from build123d import *

# Parameters (mm, degrees)
F0_W      = 1219.2
F0_H      = 50.8
F1_DEPTH  = 609.6
F3_R      = 10.16
F4_R      = 10.16
F5_R      = 10.16
F6_R      = 10.16
F7_R      = 5.08
F8_W      = 63.5
F8_H      = 63.5
F9_DEPTH  = 457.2
F10_R     = 7.62
F11_W     = 63.5
F11_H     = 63.5
F12_DEPTH = 457.2
F13_R     = 7.62
F14_W     = 63.5
F14_H     = 63.5
F15_DEPTH = 457.2
F16_R     = 7.62
F17_W     = 63.5
F17_H     = 63.5
F18_DEPTH = 457.2
F19_R     = 7.62


with BuildPart() as f1:
    # F0 (on Front) → F1 (new body)
    with BuildSketch(Plane.XZ):
        Rectangle(F0_W, F0_H)
    extrude(amount=F1_DEPTH)

    # F3
    f3_edges = [f1.edges().sort_by_distance(p)[0] for p in [
        (-609.6, -609.6, 0),
    ]]
    fillet(f3_edges, radius=F3_R)

    # F4
    f4_edges = [f1.edges().sort_by_distance(p)[0] for p in [
        (-609.6, 0, 0),
    ]]
    fillet(f4_edges, radius=F4_R)

    # F5
    f5_edges = [f1.edges().sort_by_distance(p)[0] for p in [
        (609.6, 0, 0),
    ]]
    fillet(f5_edges, radius=F5_R)

    # F6
    f6_edges = [f1.edges().sort_by_distance(p)[0] for p in [
        (609.6, -609.6, 0),
    ]]
    fillet(f6_edges, radius=F6_R)

    # F7
    f7_edges = [f1.edges().sort_by_distance(p)[0] for p in [
        (-609.6, -304.8, 25.4),
        (-609.6, -304.8, -25.4),
    ]]
    fillet(f7_edges, radius=F7_R)

    # F8 (on face) → F9 (join)
    with BuildSketch(Plane(origin=(0, 0, -25.4), x_dir=(1, 0, 0), z_dir=(0, 0, -1))):
        with Locations((-538.884262, 70.392589)):
            Rectangle(F8_W, F8_H)
    extrude(amount=F9_DEPTH)

    # F10
    f10_edges = [f1.edges().sort_by_distance(p)[0] for p in [
        (-507.134262, -38.642589, -254),
        (-507.134262, -102.142589, -254),
        (-570.634262, -102.142589, -254),
        (-570.634262, -38.642589, -254),
    ]]
    fillet(f10_edges, radius=F10_R)

    # F11 (on face) → F12 (join)
    with BuildSketch(Plane(origin=(0, 0, -25.4), x_dir=(1, 0, 0), z_dir=(0, 0, -1))):
        with Locations((533.460811, 75.974436)):
            Rectangle(F11_W, F11_H)
    extrude(amount=F12_DEPTH)

    # F13
    f13_edges = [f1.edges().sort_by_distance(p)[0] for p in [
        (565.210811, -107.724436, -254),
        (565.210811, -44.224436, -254),
        (501.710811, -107.724436, -254),
        (501.710811, -44.224436, -254),
    ]]
    fillet(f13_edges, radius=F13_R)

    # F14 (on face) → F15 (join)
    with BuildSketch(Plane(origin=(0, 0, -25.4), x_dir=(1, 0, 0), z_dir=(0, 0, -1))):
        with Locations((-538.621542, 539.01282)):
            Rectangle(F14_W, F14_H)
    extrude(amount=F15_DEPTH)

    # F16
    f16_edges = [f1.edges().sort_by_distance(p)[0] for p in [
        (-570.371542, -570.76282, -254),
        (-506.871542, -570.76282, -254),
        (-506.871542, -507.26282, -254),
        (-570.371542, -507.26282, -254),
    ]]
    fillet(f16_edges, radius=F16_R)

    # F17 (on face) → F18 (join)
    with BuildSketch(Plane(origin=(0, 0, -25.4), x_dir=(1, 0, 0), z_dir=(0, 0, -1))):
        with Locations((538.63135, 542.144825)):
            Rectangle(F17_W, F17_H)
    extrude(amount=F18_DEPTH)

    # F19
    f19_edges = [f1.edges().sort_by_distance(p)[0] for p in [
        (570.38135, -573.894825, -254),
        (506.88135, -573.894825, -254),
        (506.88135, -510.394825, -254),
        (570.38135, -510.394825, -254),
    ]]
    fillet(f19_edges, radius=F19_R)


solid = f1.part
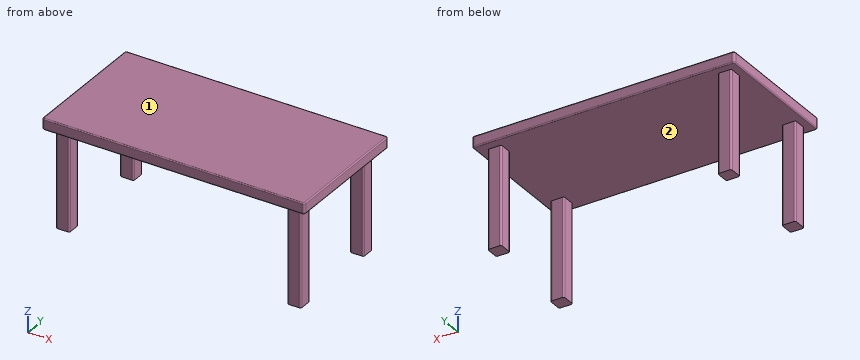
Part model, mm, in its own coordinate system. Face numbers are marked on the shaded views. A direction names the side the tool comes from. Coordinates: 2 decimals unless noted, no trailing zeros. Write each loop counter-clockwise with the first axis right and the second up, starting at its lowest first coordinate (ties: lowest second). Pieces come first, ordered by that corner, then holes. Notation, with made-up numbers: (11, -8.5) - (43, -8.5) arc R22 cw to (43, 12.5) - close; hole circle Ø2 at (35.25, 89). An arc over 180 degrees is marked (long way). Put each result on its own line as item: value.
1. Band-saw the part on A-A (z = -155.5). Give the number of separate pieces and of enclosed holes in the cut face, then the cut area to 3 significant figures.
Final values:
separate pieces: 4
enclosed holes: 0
area: 15,900 mm²
2. Flat gauge pins, fed straight in: pin 1 Ø14.5 at (x, z) = (546.5, -329) entering from -Y; pin 2 Ø24 at (x, z) = (521.5, -150) entering from +Y; pin 3 Ø14.5 at (y, z) = (-77.5, -307.5) entering from -X; pin 4 Ø10 at (y, z) = (-501, -238) entering from -X. Where does each tip first touch, or does it go through?
Final values:
pin 1: stops at y = -573.89
pin 2: stops at y = -44.22
pin 3: stops at x = -570.63
pin 4: passes through
3. 3-axis set-ups, long thin cutter, end or side, ignore diameter. For the marked faces 1 and 2: which of +Z, -Z, +X, -X, +Y, -Y reach the whole face in a straight line?
Final values:
face 1: +Z, +X, -X, +Y, -Y
face 2: -Z
4. Band-saw the part on B-B (y = -232.5). Write the cut outline in (x, z).
Final values:
outline: (-609.6, -20.32) arc R5.08 ccw to (-604.52, -25.4) - (604.52, -25.4) arc R5.08 ccw to (609.6, -20.32) - (609.6, 20.32) arc R5.08 ccw to (604.52, 25.4) - (-604.52, 25.4) arc R5.08 ccw to (-609.6, 20.32) - close
5. Probe line 1 along X through (y, z) = (-53, -279.5); line 2 along X through (y, z) = (-556.5, -399); line 3 along Z through (x, y) = (-439.5, -131). List the from-to ranges inside material, lowest first. Write a range as [from, to].
Final values:
line 1: x = [-570.63, -507.13], [501.71, 565.21]
line 2: x = [-570.37, -506.87], [506.88, 570.38]
line 3: z = [-25.4, 25.4]
6. Band-saw the part on C-C (x = -314). Write the cut outline in (y, z).
Final values:
outline: (-609.6, -20.32) arc R5.08 ccw to (-604.52, -25.4) - (-5.08, -25.4) arc R5.08 ccw to (0, -20.32) - (0, 20.32) arc R5.08 ccw to (-5.08, 25.4) - (-604.52, 25.4) arc R5.08 ccw to (-609.6, 20.32) - close
